from build123d import *

# Parameters (mm, degrees)
CROQUIS1_R              = 1.1
SALIENTE_EXTRUIR1_DEPTH = 7
CORTAR_EXTRUIR1_DEPTH   = 62.365511626
CROQUIS3_R              = 2
CORTAR_EXTRUIR3_DEPTH   = 76.80759879
CROQUIS4_R              = 3.75
CORTAR_EXTRUIR4_DEPTH   = 76.80759879
CROQUIS5_R              = 3.75
CORTAR_EXTRUIR5_DEPTH   = 76.80759879


with BuildPart() as part:
    # Croquis1 → Saliente-Extruir1 (new body)
    with BuildSketch(Plane.XY):
        Polygon((-5, 27.478679656), (-5, -5), (5, -5), (5, 27.478679656), (7.121320344, 29.6), (20.002640687, 29.6), (25, 34.597359313), (25, 47.357359313), (27.121320344, 49.478679656), (27.121320344, 52.478679656), (25, 54.6), (20, 54.6), (20, 34.6), (-20, 34.6), (-20, 54.6), (-25, 54.6), (-27.121320344, 52.478679656), (-27.121320344, 49.478679656), (-25, 47.357359313), (-25, 34.597359313), (-20.002640687, 29.6), (-7.121320344, 29.6), align=None)
        Circle(CROQUIS1_R, mode=Mode.SUBTRACT)
    extrude(amount=SALIENTE_EXTRUIR1_DEPTH)

    # Croquis2 → Cortar-Extruir1 (cut, through all)
    with BuildSketch(Plane(origin=(0, 0, 0), x_dir=(-1, 0, 0), z_dir=(0, 0, -1))):
        Polygon((-5, -5), (-2.878679656, -5), (-5, -2.878679656), align=None)
        Polygon((2.878679656, -5), (5, -2.878679656), (5, -5), align=None)
    extrude(amount=-CORTAR_EXTRUIR1_DEPTH, mode=Mode.SUBTRACT)

    # Croquis3 → Cortar-Extruir3 (cut, through all)
    with BuildSketch(Plane.ZY.offset(25)):
        with Locations(Location((3.5, 44.597359313, 0), (0, 0, 270))):
            Circle(CROQUIS3_R)
    extrude(amount=-CORTAR_EXTRUIR3_DEPTH, mode=Mode.SUBTRACT)

    # Croquis4 → Cortar-Extruir4 (cut, through all)
    with BuildSketch(Plane.ZY.offset(25)):
        with Locations((3.5, 44.597359313)):
            Circle(CROQUIS4_R)
    extrude(amount=CORTAR_EXTRUIR4_DEPTH, mode=Mode.SUBTRACT)

    # Croquis5 → Cortar-Extruir5 (cut, through all)
    with BuildSketch(Plane(origin=(25, 0, 0), x_dir=(0, 0, -1), z_dir=(1, 0, 0))):
        with Locations((-3.5, 44.597359313)):
            Circle(CROQUIS5_R)
    extrude(amount=CORTAR_EXTRUIR5_DEPTH, mode=Mode.SUBTRACT)


solid = part.part
The model under review builds one solid part; all positions refer to its coordinate system, in mm. A direction names the side the tool comes from. Coordinates: 2 decimals unless noted, no trailing zeros. Order: outer loops, then holes, each group sorted by start corner. A loop starts at its lowest first (then second) coordinate and runs counter-clockwise, first axis right, second up. Notation, with made-up numbers: (1, 26.25) -> (55, 26.25) arc R24 ccw to (55, 38.25) -> close; hole circle Ø9 at (47, -8.5). An arc over 180 degrees is marked (long way). Answer in a Markdown table with one row per item.
(1) Consider section B-B (y = 0). Write out the cut boundary in (x, z).
Answers:
| item | result |
|---|---|
| outline | (-5, 0) -> (-1.1, 0) -> (-1.1, 7) -> (-5, 7) -> close; (1.1, 0) -> (5, 0) -> (5, 7) -> (1.1, 7) -> close |
(2) Consider section C-C (z = 3.5). State how many separate pieces and enclosed holes the cut face has, plus the area to 3 significant figures.
Answers:
| item | result |
|---|---|
| separate pieces | 3 |
| enclosed holes | 1 |
| area | 748 mm² |
(3) Consider section A-A (x = 0). Write out the cut boundary in (y, z).
Answers:
| item | result |
|---|---|
| outline | (-5, 0) -> (-1.1, 0) -> (-1.1, 7) -> (-5, 7) -> close; (1.1, 0) -> (34.6, 0) -> (34.6, 7) -> (1.1, 7) -> close |
(4) Machinability: for faces 4 (the flat face through (13, 29.6, 3)), 5 (the flat face through (26.1, 53.5, 3.5)), 6 (the flat face through (0, -5, 3)), 7 (the flat face through (-14, 29.6, 3)), 8 (the flat face through (0, 34.6, 3)), which of the approach directions +Z, -Z, +X, -X, +Y, -Y give a long, thin tool a straight path to every point of the face, cutting with its end or side? Answer none if there is none.
Answers:
| item | result |
|---|---|
| face 4 | +Z, -Z, +X, -Y |
| face 5 | +Z, -Z, +X, +Y |
| face 6 | +Z, -Z, +X, -X, -Y |
| face 7 | +Z, -Z, -X, -Y |
| face 8 | +Z, -Z, +Y |
(5) Wall thickness on line 1 along X through (y, z) = (36, 5); line 2 along Y through (x, z) = (0, 1.75); line 3 along X through (y, z) = (51, 5.5): over which ranges is each line inside the solid? List them lowest first.
Answers:
| item | result |
|---|---|
| line 1 | -25 to -20, 20 to 25 |
| line 2 | -5 to -1.1, 1.1 to 34.6 |
| line 3 | -27.12 to -20, 20 to 27.12 |
(6) Consider section D-D (y = 13). Write out the cut boundary in (x, z).
Answers:
| item | result |
|---|---|
| outline | (-5, 0) -> (5, 0) -> (5, 7) -> (-5, 7) -> close |
(7) The part is to be moulded in two halves that separate along Y. For faces 1 (the cylindrical face through (22.47, 42.69, 4.1)), 2 (the flat face through (-26, 53.6, 3.5)), 3 (the flat face through (26.28, 48.64, 3.45)), say which applies: +Y half, -Y half, draft (parallel to the pull), parting line (faces both ways), or undercut.
Answers:
| item | result |
|---|---|
| face 1 | undercut |
| face 2 | +Y half |
| face 3 | -Y half |
(8) Insertion check: pin 1 (3.5 mm diameter, centred on y = 45, z = 4.5, fed in from +X); pin 2 (2 mm diameter, centred on y = 38.5, z = 5, fed in from -X); pin 3 (3 mm diameter, centred on y = 19, z = 6, fed in from +X). Each pin has a flat end and moves straight along its axis. Give the tip position at first contact, or say it passes through.
Answers:
| item | result |
|---|---|
| pin 1 | x = 25 |
| pin 2 | x = -25 |
| pin 3 | x = 5 |
